The model under review builds one solid part; all positions refer to its coordinate system, in mm. Face numbers are marked on the shaded views. A direction names the side the tool comes from. Coordinates: 2 decimals unless noted, no trailing zeros. Loops run counter-clockwise (first coordinate to the right, second up) from the corner with the lowest first, then second, coordinate; pieces in that order, holes last. Notation, with made-up numbers: (26, 74.25) - (61, 74.25) arc R21 ccw to (61, 91.25) - close; hole circle Ø5 at (56.5, 60). An arc over 180 degrees is marked (long way). Use a Markdown table: item, result. Add a question column.
1) The part is to be moulded in two halves that separate along Y. For the marked faces 4, 5 and 6, say which applies: pulls with the +Y half, pulls with the -Y half, needs draft (parallel to the pull), parting line crosses it, or undercut.
2) To check wall thickness, follow L1, parallel to Z at x = 1.25, y = 2.25; L2, parallel to X at y = 1, z = -5.25. State the ranges of each line that lie inside material, in increasing order. Write a range as [from, to].
3) Add section A-A, the plane z = -9.5. Give the boundary of the cut face in (x, y).
4) For the marked faces 1, 2 and 3, list the 3-axis set-ups (+Z, -Z, +X, -X, +Y, -Y) from which the entire face can be reached by the end or side of a thin tool; tool diameter is ignored.
5) Clearance check with a flat-ended pin moving along its axis: pin 1 (1.5 mm diameter, centred on y = 2, z = -7, fed in from +X). State where the tip first meets the part, or that it passes through.
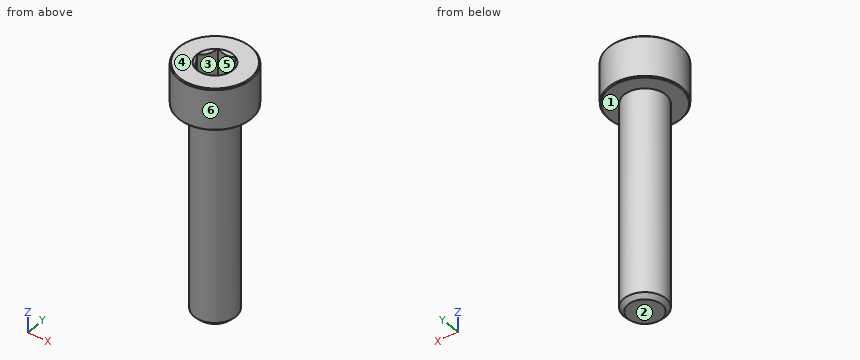
```python
from build123d import *

# Parameters (mm, degrees)
SKETCH001_R     = 3.75
POCKET_DEPTH    = 9.70192
CHAMFER_SIZE    = 0.4
CHAMFER001_SIZE = 0.1
CHAMFER002_SIZE = 0.4


with BuildPart() as pocket:
    # Sketch003 → Revolution001 (revolve)
    with BuildSketch(Plane.XZ):
        Polygon((0, 0.29908), (2.75, 1.3), (2.75, 10), (0, 10), align=None)
    revolve(axis=Axis((0, 0, 0), (0, 0, 1)))

    # Sketch001 → Pocket (cut, through all)
    with BuildSketch(Plane(origin=(0, 0, 10), x_dir=(-1, 0, 0), z_dir=(0, 0, 1))):
        Circle(SKETCH001_R)
        Polygon((-0.866025, 1.5), (0.866025, 1.5), (1.732051, 0), (0.866025, -1.5), (-0.866025, -1.5), (-1.732051, 0), align=None, mode=Mode.SUBTRACT)
    extrude(amount=-POCKET_DEPTH, mode=Mode.SUBTRACT)


with BuildPart() as chamfer002:
    # Sketch → Revolution (revolve)
    with BuildSketch(Plane.XZ):
        Polygon((1.73, 4), (3.5, 4), (3.5, 0), (2, 0), (2, -20), (0, -20), (0, 2.269998), align=None)
    revolve(axis=Axis((0, 0, 0), (0, 0, 1)))

    # Cut: cut Pocket
    add(pocket.part, mode=Mode.SUBTRACT)

    # Chamfer
    chamfer_edges = [chamfer002.edges().sort_by_distance(p)[0] for p in [
        (1.299038, 0.75, 0.845037),
    ]]
    chamfer(chamfer_edges, length=CHAMFER_SIZE)

    # Chamfer001
    chamfer001_edges = [chamfer002.edges().sort_by_distance(p)[0] for p in [
        (-3.5, 0, 4),
        (-3.5, 0, 0),
    ]]
    chamfer(chamfer001_edges, length=CHAMFER001_SIZE)

    # Chamfer002
    chamfer002_edges = [chamfer002.edges().sort_by_distance(p)[0] for p in [
        (-2, 0, -20),
    ]]
    chamfer(chamfer002_edges, length=CHAMFER002_SIZE)


solid = chamfer002.part
```
From the geometry:
| question | item | result |
|---|---|---|
| 1 | face 4 | needs draft |
| 1 | face 5 | undercut |
| 1 | face 6 | parting line crosses it |
| 2 | L1 | z = [0, 4] |
| 2 | L2 | x = [-1.73, 1.73] |
| 3 | outline | circle Ø4 at (0, 0) |
| 4 | face 1 | -Z |
| 4 | face 2 | -Z, +X, -X, +Y, -Y |
| 4 | face 3 | +Z |
| 5 | pin 1 | stops at x = 1.56 |
